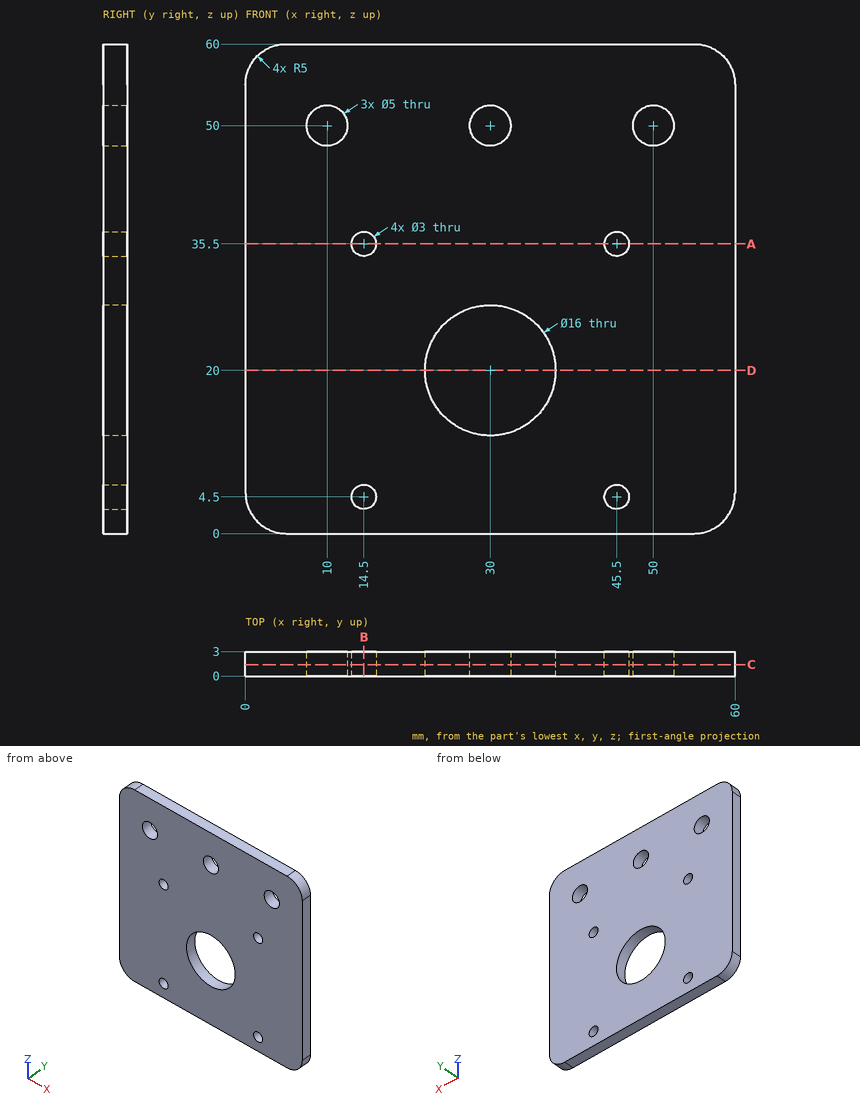
Answer from the drawing. Dimensions are ordinates in mm from the lowest x, y and z of the part. Give positions to 0.01 mm unless a question says otherwise; leave off trailing zeros. Loops run counter-clockwise (first coordinate to the right, second up) from the corner with the lowest first, then second, coordinate; pieces in that order, holes last. Notation, with made-up numbers: M 73,-11.75 L 112,-11.75 A34 ccw 112,23.25 Z; hole C -6,64.25 d5. An arc over 180 degrees is marked long. One line per item, written item: value.
Q1. A cutting plane is placed at C-C on y = 1.4. Give the number of separate pieces and of enclosed holes in the cut face, then the cut area to 3 significant figures.
Working result:
separate pieces: 1
enclosed holes: 8
area: 3,290 mm^2
Q2. A cutting plane is placed at D-D on z = 20. Determine the outline of the cut face in (x, y).
Working result:
outline: M 0,0 L 22,0 L 22,3 L 0,3 Z; M 38,0 L 60,0 L 60,3 L 38,3 Z
Q3. A cutting plane is placed at B-B on x = 14.5. Determine the outline of the cut face in (y, z), then the cut area to 3 significant figures.
Working result:
outline: M 0,0 L 3,0 L 3,3 L 0,3 Z; M 0,6 L 3,6 L 3,34 L 0,34 Z; M 0,37 L 3,37 L 3,60 L 0,60 Z
area: 162 mm^2
Q4. A flat-ended cylindrical pin translates along its axis: P1, Ø13, axis at x = 30, z = 20, coming from the +Y side. Find the tip coordinate at first contact, or state that the pin passes through.
Working result:
P1: passes through
Q5. Find the intervals of material crossed by line 1 (Z direction, x = 30, y = 2.4); line 2 (X direction, y = 1.6, z = 50); line 3 (X direction, y = 1, z = 35.5), in increasing order. Write a range as from..to.
Working result:
line 1: z = 0..12, 28..47.5, 52.5..60
line 2: x = 0..7.5, 12.5..27.5, 32.5..47.5, 52.5..60
line 3: x = 0..13, 16..44, 47..60
Q6. A cutting plane is placed at A-A on z = 35.5. Determine the outline of the cut face in (x, y).
Working result:
outline: M 0,0 L 13,0 L 13,3 L 0,3 Z; M 16,0 L 44,0 L 44,3 L 16,3 Z; M 47,0 L 60,0 L 60,3 L 47,3 Z
